```python
from build123d import *

# Parameters (mm, degrees)
F1_DEPTH = 8
F2_DEPTH = 25


with BuildPart() as f1:
    # F0 (on Top) → F1 (new body)
    with BuildSketch(Plane.XY):
        with BuildLine():
            Line((-49.977526, -41.605607), (-58.697784, -50.980339))
            ThreePointArc((-58.697784, -50.980339), (-55.746943, -49.98082), (-52.693043, -49.364224))
            ThreePointArc((-52.693043, -49.364224), (-47.439924, -53.121601), (-44.515088, -58.879941))
            Line((-44.515088, -58.879941), (-35.81804, -52.855607))
            Line((-35.81804, -52.855607), (-28.059421, -60.42026))
            Line((-28.059421, -60.42026), (-16.80702, -52.855607))
            Line((-16.80702, -52.855607), (-8.662867, -62.359914))
            Line((-8.662867, -62.359914), (0, -54.936784))
            Line((0, -54.936784), (8.631467, -63.911639))
            ThreePointArc((8.631467, -63.911639), (11.744426, -54.491495), (20.237995, -49.364224))
            ThreePointArc((20.237995, -49.364224), (23.355468, -50.303762), (26.277462, -51.740186))
            Line((26.277462, -51.740186), (20.237995, -43.545261))
            Line((20.237995, -43.545261), (20.237995, -37.920259))
            Line((20.237995, -37.920259), (28.72714, -30.080417))
            ThreePointArc((28.72714, -30.080417), (43.074733, 13.306863), (24.342671, 54.989226))
            ThreePointArc((24.342671, 54.989226), (-9.855567, 68.032469), (-44.127155, 55.183191))
            ThreePointArc((-44.127155, 55.183191), (-65.822797, 15.690348), (-58.705974, -28.803879))
            Line((-58.705974, -28.803879), (-49.977526, -35.010777))
            Line((-49.977526, -35.010777), (-49.977526, -41.605607))
        make_face()
        Polygon((0, -16.390087), (-21.627156, -16.390087), (-9.989223, 0), align=None, mode=Mode.SUBTRACT)
        with BuildLine():
            ThreePointArc((-26.282329, 25.894396), (-41.063186, 22.944871), (-42.769399, 37.920259))
            Line((-42.769399, 37.920259), (-26.282329, 25.894396))
        make_face(mode=Mode.SUBTRACT)
        with BuildLine():
            ThreePointArc((14.450433, 38.696121), (14.608633, 23.960948), (0, 25.894396))
            Line((0, 25.894396), (14.450433, 38.696121))
        make_face(mode=Mode.SUBTRACT)
    extrude(amount=F1_DEPTH)

    # F0 (on Top) → F2 (join)
    with BuildSketch(Plane.XY):
        with BuildLine():
            ThreePointArc((-54.989226, -57.375513), (-61.534535, -55.666613), (-67.984916, -57.704747))
            ThreePointArc((-67.984916, -57.704747), (-58.884264, -69.778136), (-44.515088, -65.075435))
            ThreePointArc((-44.515088, -65.075435), (-48.164701, -59.06607), (-54.989226, -57.375513))
        make_face()
        with BuildLine():
            ThreePointArc((-58.697784, -50.980339), (-63.740644, -53.791075), (-67.984916, -57.704747))
            ThreePointArc((-67.984916, -57.704747), (-61.534535, -55.666613), (-54.989226, -57.375513))
            ThreePointArc((-54.989226, -57.375513), (-48.164701, -59.06607), (-44.515088, -65.075435))
            ThreePointArc((-44.515088, -65.075435), (-44.157255, -61.977688), (-44.515088, -58.879941))
            ThreePointArc((-44.515088, -58.879941), (-47.439924, -53.121601), (-52.693043, -49.364224))
            ThreePointArc((-52.693043, -49.364224), (-55.746943, -49.98082), (-58.697784, -50.980339))
        make_face()
        with BuildLine():
            Line((-49.977526, -41.605607), (-58.697784, -50.980339))
            ThreePointArc((-58.697784, -50.980339), (-55.746943, -49.98082), (-52.693043, -49.364224))
            ThreePointArc((-52.693043, -49.364224), (-47.439924, -53.121601), (-44.515088, -58.879941))
            Line((-44.515088, -58.879941), (-35.81804, -52.855607))
            Line((-35.81804, -52.855607), (-28.059421, -60.42026))
            Line((-28.059421, -60.42026), (-16.80702, -52.855607))
            Line((-16.80702, -52.855607), (-8.662867, -62.359914))
            Line((-8.662867, -62.359914), (0, -54.936784))
            Line((0, -54.936784), (8.631467, -63.911639))
            ThreePointArc((8.631467, -63.911639), (11.744426, -54.491495), (20.237995, -49.364224))
            ThreePointArc((20.237995, -49.364224), (23.355468, -50.303762), (26.277462, -51.740186))
            Line((26.277462, -51.740186), (20.237995, -43.545261))
            Line((20.237995, -43.545261), (20.237995, -37.920259))
            Line((20.237995, -37.920259), (28.72714, -30.080417))
            ThreePointArc((28.72714, -30.080417), (43.074733, 13.306863), (24.342671, 54.989226))
            ThreePointArc((24.342671, 54.989226), (-9.855567, 68.032469), (-44.127155, 55.183191))
            ThreePointArc((-44.127155, 55.183191), (-65.822797, 15.690348), (-58.705974, -28.803879))
            Line((-58.705974, -28.803879), (-49.977526, -35.010777))
            Line((-49.977526, -35.010777), (-49.977526, -41.605607))
        make_face()
        Polygon((0, -16.390087), (-21.627156, -16.390087), (-9.989223, 0), align=None, mode=Mode.SUBTRACT)
        with BuildLine():
            ThreePointArc((-26.282329, 25.894396), (-41.063186, 22.944871), (-42.769399, 37.920259))
            Line((-42.769399, 37.920259), (-26.282329, 25.894396))
        make_face(mode=Mode.SUBTRACT)
        with BuildLine():
            ThreePointArc((14.450433, 38.696121), (14.608633, 23.960948), (0, 25.894396))
            Line((0, 25.894396), (14.450433, 38.696121))
        make_face(mode=Mode.SUBTRACT)
        with BuildLine():
            ThreePointArc((22.355094, -58.863486), (14.893383, -59.756716), (8.631467, -63.911639))
            ThreePointArc((8.631467, -63.911639), (21.724486, -73.472528), (35.592671, -65.075435))
            ThreePointArc((35.592671, -65.075435), (29.710772, -60.399159), (22.355094, -58.863486))
        make_face()
        with BuildLine():
            ThreePointArc((20.237995, -49.364224), (11.744426, -54.491495), (8.631467, -63.911639))
            ThreePointArc((8.631467, -63.911639), (14.893383, -59.756716), (22.355094, -58.863486))
            ThreePointArc((22.355094, -58.863486), (29.710772, -60.399159), (35.592671, -65.075435))
            ThreePointArc((35.592671, -65.075435), (32.363421, -57.410047), (26.277462, -51.740186))
            ThreePointArc((26.277462, -51.740186), (23.355468, -50.303762), (20.237995, -49.364224))
        make_face()
    extrude(amount=F2_DEPTH)


solid = f1.part
```
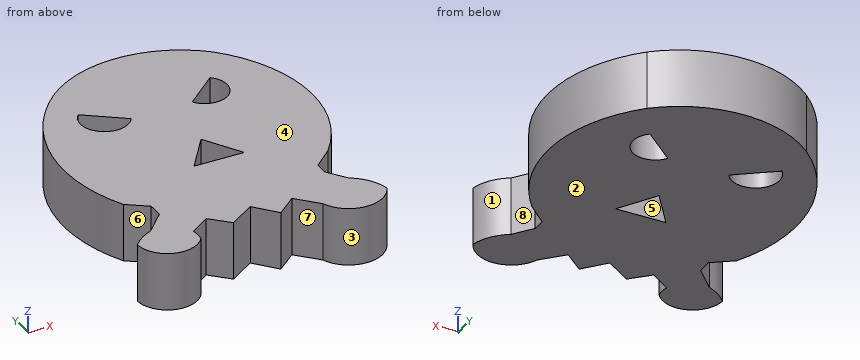
Here's how the part is built. I have some questions about the finished solid (model axes, mm). Face numbers are marked on the shaded views. A direction names the side the tool comes from. Give positions to 0.01 mm unless a question says otherwise; leave off trailing zeros. Write each loop counter-clockwise with the first axis right and the second up, starting at its lowest first coordinate (ties: lowest second). Pieces come first, ordered by that corner, then holes.
(1) Will these pins go through, and if not, where does the flat tip stop? pin 1 (12 mm diameter, centred on y = -38.5, z = 11, fed in from -X); pin 2 (5 mm diameter, centred on x = -8.5, z = 14.5, fed in from +Y); pin 3 (5.5 mm diameter, centred on y = -39, z = 17, fed in from -X).
Output values:
pin 1: stops at x = -53.51
pin 2: stops at y = 68.03
pin 3: stops at x = -50.11
(2) On a 3-axis mill with a long thin cutter (end or side, diameter ignored), from which of +Z, -Z, +X, -X, +Y, -Y can I reach the whole of each face in a straight line? I mean the marked faces 4, 5, 6, 7 and 8. Say none if no direction works.
Output values:
face 4: +Z, +X, -X, +Y, -Y
face 5: +Z, -Z
face 6: +Z, -Z, -X
face 7: +Z, -Z, -Y
face 8: +Z, -Z, +X
(3) Imagine slicing it at D-D, the plane y = 24. Write out the boundary of the cut face in (x, z), and give its area (3 significant figures).
Output values:
outline: (-63.85, 0) - (-42.29, 0) - (-42.29, 25) - (-63.85, 25) - close; (-27.77, 0) - (1.63, 0) - (1.63, 25) - (-27.77, 25) - close; (14.65, 0) - (41.6, 0) - (41.6, 25) - (14.65, 25) - close
area: 1,950 mm2
(4) Imagine slicing it at A-A, the plane z = 19.75. Write out the boundary of the cut face in (x, y).
Output values:
outline: (-67.98, -57.7) arc R13 ccw to (-44.52, -65.08) arc R13.59 ccw to (-44.52, -58.88) - (-35.82, -52.86) - (-28.06, -60.42) - (-16.81, -52.86) - (-8.66, -62.36) - (0, -54.94) - (8.63, -63.91) arc R14.62 ccw to (35.59, -65.08) arc R19.85 ccw to (26.28, -51.74) - (20.24, -43.55) - (20.24, -37.92) - (28.73, -30.08) arc R63.05 ccw to (24.34, 54.99) arc R51.74 ccw to (-44.13, 55.18) arc R69.43 ccw to (-58.71, -28.8) - (-49.98, -35.01) - (-49.98, -41.61) - (-58.7, -50.98) arc R24.48 ccw to start; hole (-42.77, 37.92) arc R10.24 ccw (long way) to (-26.28, 25.89) - close; hole (-21.63, -16.39) - (0, -16.39) - (-9.99, 0) - close; hole (0, 25.89) arc R9.75 ccw (long way) to (14.45, 38.7) - close
(5) If I drill on L1, parallel to X at y = -61.5, z = 14.5; L2, parallel to Y at x = -21, z = 9; L3, parallel to X at y = 29.5, z = 5.5, over which ranges is the centre line in solid material (lowest first)?
Output values:
L1: x = -67.32 to -44.17, -9.4 to -7.66, 6.31 to 34.56
L2: y = -55.67 to -16.39, -15.51 to 66.85
L3: x = -61.92 to -45.12, -31.23 to 4.07, 17.73 to 40.09
(6) Thinking about a two-plate mould opening in X: for the marked faces 1, 2 and 3, which applies, pulls with the +X half, pulls with the -X half, needs draft (parallel to the pull), parting line crosses it, or undercut?
Output values:
face 1: pulls with the +X half
face 2: needs draft
face 3: undercut
(7) Imagine slicing it at B-B, the plane y = -2.5. Write out the boundary of the cut face in (x, z).
Output values:
outline: (-66.56, 0) - (-11.76, 0) - (-11.76, 25) - (-66.56, 25) - close; (-8.47, 0) - (41.89, 0) - (41.89, 25) - (-8.47, 25) - close
(8) Imagine slicing it at C-C, the plane x = -38. Write out the boundary of the cut face in (y, z), and give its area (3 significant figures).
Output values:
outline: (-54.37, 0) - (21.42, 0) - (21.42, 25) - (-54.37, 25) - close; (34.44, 0) - (59.8, 0) - (59.8, 25) - (34.44, 25) - close
area: 2,530 mm2
